from build123d import *

# Parameters (mm, degrees)
BOSS_EXTRUDE6_DEPTH   = 3
BOSS_EXTRUDE6_2_DEPTH = 3
SKETCH4_W             = 119.7
SKETCH4_H             = 55
BOSS_EXTRUDE7_DEPTH   = 1
FILLET13_R            = 3
FILLET14_R            = 1
FILLET15_R            = 1
FILLET16_R            = 3
FILLET17_R            = 3
FILLET18_R            = 1
FILLET19_R            = 3
FILLET20_R            = 1


with BuildPart() as part:
    # Sketch3 → Boss-Extrude6 (new body)
    with BuildSketch(Plane(origin=(0, 0, 0), x_dir=(1, 0, 0), z_dir=(0, 1, 0))):
        Polygon((-35.6, -27.5), (-59.85, -27.5), (-59.85, 27.5), (-35.6, 27.5), (-35.6, 42.5), (-37.6, 42.5), (-37.6, 30.5), (-62.85, 30.5), (-62.85, -30.5), (-37.6, -30.5), (-37.6, -42.5), (-35.6, -42.5), align=None)
    extrude(amount=BOSS_EXTRUDE6_DEPTH)



with BuildPart() as body_2:
    # Sketch3 → Boss-Extrude6 2 (new body)
    with BuildSketch(Plane(origin=(0, 0, 0), x_dir=(1, 0, 0), z_dir=(0, 1, 0))):
        Polygon((59.85, -27.5), (-4.4, -27.5), (-4.4, -42.5), (-2.4, -42.5), (-2.4, -30.5), (62.85, -30.5), (62.85, 30.5), (-2.4, 30.5), (-2.4, 42.5), (-4.4, 42.5), (-4.4, 27.5), (59.85, 27.5), align=None)
    extrude(amount=BOSS_EXTRUDE6_2_DEPTH)


with BuildPart() as part_1:
    add(part.part)

    add(body_2.part)  # Boss-Extrude7 merges body 2
    # Sketch4 → Boss-Extrude7 (add)
    with BuildSketch(Plane(origin=(0, 0, 0), x_dir=(1, 0, 0), z_dir=(0, 1, 0))):
        Rectangle(SKETCH4_W, SKETCH4_H)
    extrude(amount=BOSS_EXTRUDE7_DEPTH)

    # Fillet13
    fillet13_edges = [part_1.edges().sort_by_distance(p)[0] for p in [
        (-62.85, 1.5, 30.5),
        (-62.85, 1.5, -30.5),
        (62.85, 1.5, 30.5),
        (62.85, 1.5, -30.5),
    ]]
    fillet(fillet13_edges, radius=FILLET13_R)

    # Fillet14
    fillet14_edges = [part_1.edges().sort_by_distance(p)[0] for p in [
        (-59.85, 2, -27.5),
        (-59.85, 2, 27.5),
        (59.85, 2, -27.5),
        (59.85, 2, 27.5),
    ]]
    fillet(fillet14_edges, radius=FILLET14_R)

    # Fillet15
    fillet15_edges = [part_1.edges().sort_by_distance(p)[0] for p in [
        (-2.4, 1.5, 42.5),
        (-4.4, 1.5, 42.5),
        (-35.6, 1.5, 42.5),
        (-37.6, 1.5, 42.5),
        (-35.6, 1.5, -42.5),
        (-37.6, 1.5, -42.5),
        (-2.4, 1.5, -42.5),
        (-4.4, 1.5, -42.5),
    ]]
    fillet(fillet15_edges, radius=FILLET15_R - 0.0001)  # a hair under: the kernel refuses the full size

    # Fillet16
    fillet16_edges = [part_1.edges().sort_by_distance(p)[0] for p in [
        (-37.6, 1.5, -30.5),
        (-37.6, 1.5, 30.5),
        (-2.4, 1.5, 30.5),
        (-2.4, 1.5, -30.5),
    ]]
    fillet(fillet16_edges, radius=FILLET16_R)

    # Fillet17
    fillet17_edges = [part_1.edges().sort_by_distance(p)[0] for p in [
        (-35.6, 2, -27.5),
        (-4.4, 2, -27.5),
    ]]
    fillet(fillet17_edges, radius=FILLET17_R)

    # Fillet18
    fillet18_edges = [part_1.edges().sort_by_distance(p)[0] for p in [
        (-35.6, 0.5, -27.5),
        (-4.4, 0.5, -27.5),
    ]]
    fillet(fillet18_edges, radius=FILLET18_R)

    # Fillet19
    fillet19_edges = [part_1.edges().sort_by_distance(p)[0] for p in [
        (-35.6, 2, 27.5),
        (-4.4, 2, 27.5),
    ]]
    fillet(fillet19_edges, radius=FILLET19_R)

    # Fillet20
    fillet20_edges = [part_1.edges().sort_by_distance(p)[0] for p in [
        (-35.6, 0.5, 27.5),
        (-4.4, 0.5, 27.5),
    ]]
    fillet(fillet20_edges, radius=FILLET20_R)


solid = part_1.part
Verification items for the finished model (mm, model axes). A direction names the side the tool comes from. Coordinates: 2 decimals unless noted, no trailing zeros. Loops run counter-clockwise (first coordinate to the right, second up) from the corner with the lowest first, then second, coordinate; pieces in that order, holes last. Notation, with made-up numbers: (69, 46) -> (116, 46) arc R8 ccw to (116, 61) -> close; hole circle Ø11 at (76, -22). An arc over 180 degrees is marked (long way). Answer as a JSON object with one key per item and string values. Group by question number.
Item 1: Sectioned sample at A-A on z = 36.5. Record the boundary of the cut face in (x, y).
Item 2: Sectioned sample at D-D on x = -16. Record the boundary of the cut face in (y, z).
Item 3: Mould release check, pull along X, two halves, no side actions. Record for faces 6 (the flat face through (-2.4, 1, -37)), 7 (the flat face through (-62.85, 1, 0)), 8 (the flat face through (-4.4, 1, 35)), 9 (the flat face through (-35.6, 1, -35)): +X half, -X half, draft (parallel to the pull), parting line (faces both ways), or undercut.
Item 4: Tool access check on faces 1 (the flat face through (-37.6, 1, -38)), 2 (the flat face through (31, 1, -30.5)), 3 (the flat face through (62.85, 1, 0)), 4 (the flat face through (-35.6, 1, 35)), 5 (the cylindrical face through (-36.46, 2.01, -28.4)). Record the directions out of +Z, -Z, +X, -X, +Y, -Y that give a thin tool (end or side, any length) a straight path to the whole face; none if there is none.
Item 5: Depth check by flat-ended pin: pin 1 (0.9 mm diameter, centred on y = 2, z = 34, fed in from -X); pin 2 (1 mm diameter, centred on x = 1, z = 10.5, fed in from -Y); pin 3 (1 mm diameter, centred on x = 19, y = 1, fed in from -Z); pin 4 (0.9 mm diameter, centred on x = -54.5, y = 2, fed in from +Z). Enter the tip coordinate at first touch or a pass-through.
Item 6: Scan lines: probe 1 along X at (y, z) = (0.5, 38); probe 2 along Z at (x, y) = (23, 2.6); probe 3 along X at (y, z) = (1.8, 22.5). Record each from-to range of solid material in increasing order.
Item 7: Sectioned sample at C-C on z = 9. Record the boundary of the cut face in (x, y), plus the area to 3 significant figures.
Item 8: Sectioned sample at B-B on x = -46. Record the boundary of the cut face in (y, z), plus the area to 3 significant figures.
Evaluation:
{
 "1": {"outline": "(-37.6, 0) -> (-35.6, 0) -> (-35.6, 3) -> (-37.6, 3) -> close; (-4.4, 0) -> (-2.4, 0) -> (-2.4, 3) -> (-4.4, 3) -> close"},
 "2": {"outline": "(0, -27.5) -> (1, -27.5) -> (1, 27.5) -> (0, 27.5) -> close"},
 "3": {"face 6": "+X half", "face 7": "-X half", "face 8": "undercut", "face 9": "undercut"},
 "4": {"face 1": "-Z, -X, +Y, -Y", "face 2": "-Z, +X, +Y, -Y", "face 3": "+Z, -Z, +X, +Y, -Y", "face 4": "+Z, +Y, -Y", "face 5": "+Y"},
 "5": {"pin 1": "stops at x = -37.6", "pin 2": "stops at y = 0", "pin 3": "stops at z = -30.5", "pin 4": "stops at z = 30.5"},
 "6": {"probe 1": "x = -37.6 to -35.6, -4.4 to -2.4", "probe 2": "z = -30.5 to -27.5, 27.5 to 30.5", "probe 3": "x = -62.85 to -59.85, 59.85 to 62.85"},
 "7": {"outline": "(-62.85, 0) -> (62.85, 0) -> (62.85, 3) -> (59.85, 3) -> (59.85, 1) -> (-59.85, 1) -> (-59.85, 3) -> (-62.85, 3) -> close", "area": "138 mm²"},
 "8": {"outline": "(0, -30.5) -> (3, -30.5) -> (3, -27.5) -> (1, -27.5) -> (1, 27.5) -> (3, 27.5) -> (3, 30.5) -> (0, 30.5) -> close", "area": "73.0 mm²"}
}
